Geometry: final body of the model. Coordinates: model frame, mm. Face numbers are marked on the shaded views. A direction names the side the tool comes from. Give positions to 0.01 mm unless a question says otherwise; leave off trailing zeros. Write each loop counter-clockwise with the first axis right and the second up, starting at its lowest first coordinate (ties: lowest second). Pieces come first, ordered by that corner, then holes.
Q1. Draft query along Z for the marked faces 3, 4 and 5. Return one class per face: pulls with the +Z half, pulls with the -Z half, needs draft (parallel to the pull), parting line crosses it, or undercut.
Q2. Cut plane A-A on x = 0. Return the cut outline in (y, z).
Q3. Cut plane B-B on x = 7.5. Return the cut outline in (y, z).
Q4. Cut plane C-C on y = 9.5. Return the cut outline in (x, z), plus the area to 3 significant figures.
Q5. Reachability of the marked faces 1 and 2 from +Z, -Z, +X, -X, +Y, -Y: full face, straight path, thin tool, end or side. Return the list, or none.
Q6. Pin query (flat end, axial travel): pin 1 (1 mm diameter, centred on x = 5.5, y = -0.5, fed in from -Z); pin 2 (4.5 mm diameter, centred on x = 0, y = -9.5, fed in from -Z); pin 3 (11.5 mm diameter, centred on x = 0, y = -6.5, fed in from +Z); pin 4 (7.5 mm diameter, centred on x = 0, y = 9.5, fed in from +Z). Return the tip coordinate at first contact, or that it passes through.
Q7. Cut plane D-D on z = 1. Return the cut outline in (x, y), plus the area to 3 significant figures.
Q8. Line query: L1, parallel to Y at x = 0, z = 0.6; L2, parallel to Y at x = 0, z = 6.15; L3, parallel to X at y = -2.5, z = 11.5. Output: solid intervals per line, ascending.
```python
from build123d import *

# Parameters (mm, degrees)
F0_W     = 23
F0_H     = 32.5
F0_R     = 2.75
F1_DEPTH = 7.5
F2_R     = 4.75
F3_DEPTH = 5.5
F4_W     = 2
F4_H     = 21
F5_DEPTH = 3.5
F6_W     = 5
F6_H     = 21
F7_DEPTH = 2


with BuildPart() as f1:
    # F0 (on Top) → F1 (new body)
    with BuildSketch(Plane.XY):
        Rectangle(F0_W, F0_H)
        with Locations((0, -9.5)):
            Circle(F0_R, mode=Mode.SUBTRACT)
        with Locations((0, 9.5)):
            Circle(F0_R, mode=Mode.SUBTRACT)
    extrude(amount=F1_DEPTH)

    # F2 (on face) → F3 (cut)
    with BuildSketch(Plane.XY.offset(7.5)):
        with Locations((0, -9.5)):
            Circle(F2_R)
        with Locations((0, 9.5)):
            Circle(F2_R)
    extrude(amount=-F3_DEPTH, mode=Mode.SUBTRACT)

    # F4 (on face) → F5 (join)
    with BuildSketch(Plane.XY.offset(7.5)):
        with Locations((-10.5, -5.75)):
            Rectangle(F4_W, F4_H)
        with Locations((10.5, -5.75)):
            Rectangle(F4_W, F4_H)
    extrude(amount=F5_DEPTH)

    # F6 (on face) → F7 (join)
    with BuildSketch(Plane.XY.offset(11)):
        with Locations((-9, -5.75)):
            Rectangle(F6_W, F6_H)
        with Locations((9, -5.75)):
            Rectangle(F6_W, F6_H)
    extrude(amount=F7_DEPTH)


solid = f1.part
```
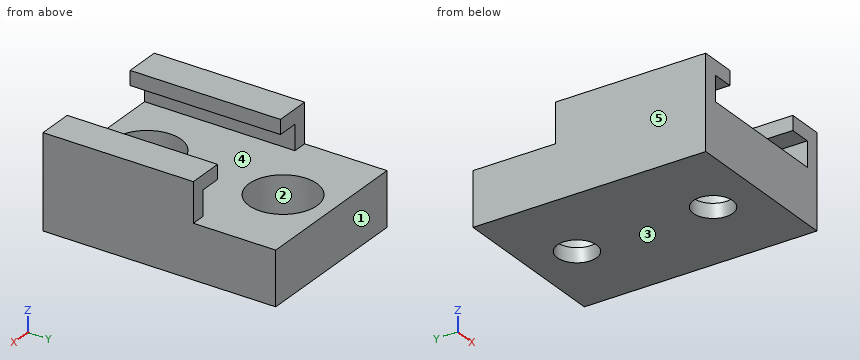
Data:
1. face 3: pulls with the -Z half
1. face 4: undercut
1. face 5: needs draft
2. outline: (-16.25, 0) - (-12.25, 0) - (-12.25, 2) - (-14.25, 2) - (-14.25, 7.5) - (-16.25, 7.5) - close; (-6.75, 0) - (6.75, 0) - (6.75, 2) - (4.75, 2) - (4.75, 7.5) - (-4.75, 7.5) - (-4.75, 2) - (-6.75, 2) - close; (12.25, 0) - (16.25, 0) - (16.25, 7.5) - (14.25, 7.5) - (14.25, 2) - (12.25, 2) - close
3. outline: (-16.25, 0) - (16.25, 0) - (16.25, 7.5) - (-16.25, 7.5) - close; (-16.25, 11) - (4.75, 11) - (4.75, 13) - (-16.25, 13) - close
4. outline: (-11.5, 0) - (-2.75, 0) - (-2.75, 2) - (-4.75, 2) - (-4.75, 7.5) - (-11.5, 7.5) - close; (2.75, 0) - (11.5, 0) - (11.5, 7.5) - (4.75, 7.5) - (4.75, 2) - (2.75, 2) - close
4. area: 109 mm2
5. face 1: +Z, -Z, +X, -X, +Y
5. face 2: +Z
6. pin 1: stops at z = 0
6. pin 2: passes through
6. pin 3: stops at z = 7.5
6. pin 4: stops at z = 2
7. outline: (-11.5, -16.25) - (11.5, -16.25) - (11.5, 16.25) - (-11.5, 16.25) - close; hole circle Ø5.5 at (0, -9.5); hole circle Ø5.5 at (0, 9.5)
7. area: 700 mm2
8. L1: y = -16.25 to -12.25, -6.75 to 6.75, 12.25 to 16.25
8. L2: y = -16.25 to -14.25, -4.75 to 4.75, 14.25 to 16.25
8. L3: x = -11.5 to -6.5, 6.5 to 11.5
